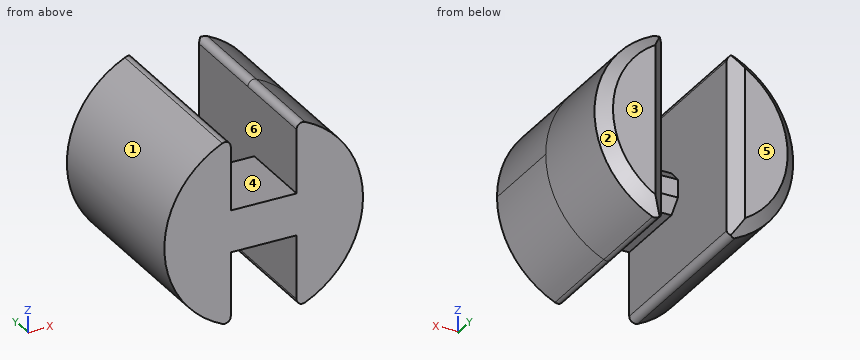
```python
from build123d import *

# Parameters (mm, degrees)
SKETCH1_W           = 2.75
SKETCH1_H           = 1.75
BOSS_EXTRUDE1_DEPTH = 3.75
BOSS_EXTRUDE2_DEPTH = 4.25
FILLET1_R           = 0.25
CHAMFER1_SIZE       = 0.5


with BuildPart() as part:
    # Sketch1 → Boss-Extrude1 (new body)
    with BuildSketch(Plane(origin=(0, 0, 0), x_dir=(1, 0, 0), z_dir=(0, 1, 0))):
        with BuildLine():
            Line((-1.375, 0.875), (-1.375, 3.915593825))
            ThreePointArc((-1.375, 3.915593825), (-4.15, 0), (-1.375, -3.915593825))
            Line((-1.375, -3.915593825), (-1.375, -0.875))
            Line((-1.375, -0.875), (-1.375, 0.875))
        make_face()
        with BuildLine():
            ThreePointArc((4.15, 0), (3.385908298, 2.399609343), (1.375, 3.915593825))
            Line((1.375, 3.915593825), (1.375, 0.875))
            Line((1.375, 0.875), (1.375, -0.875))
            Line((1.375, -0.875), (1.375, -3.915593825))
            ThreePointArc((1.375, -3.915593825), (3.385908298, -2.399609343), (4.15, 0))
        make_face()
        Rectangle(SKETCH1_W, SKETCH1_H)
    extrude(amount=BOSS_EXTRUDE1_DEPTH)

    # Sketch2 → Boss-Extrude2 (add)
    with BuildSketch(Plane(origin=(0, 3.75, 0), x_dir=(1, 0, 0), z_dir=(0, 1, 0))):
        with BuildLine():
            Line((1.375, -0.875), (1.375, 0.875))
            Line((1.375, 0.875), (1.375, 3.915593825))
            ThreePointArc((1.375, 3.915593825), (4.15, 0), (1.375, -3.915593825))
            Line((1.375, -3.915593825), (1.375, -0.875))
        make_face()
        with BuildLine():
            Line((-1.375, 0.875), (-1.375, -0.875))
            Line((-1.375, -0.875), (-1.375, -3.915593825))
            ThreePointArc((-1.375, -3.915593825), (-4.15, 0), (-1.375, 3.915593825))
            Line((-1.375, 3.915593825), (-1.375, 0.875))
        make_face()
    extrude(amount=BOSS_EXTRUDE2_DEPTH)

    # Fillet1
    fillet1_edges = [part.edges().sort_by_distance(p)[0] for p in [
        (1.375, 4, -3.915593825),
        (1.375, 4, 3.915593825),
        (-1.375, 4, 3.915593825),
        (-1.375, 4, -3.915593825),
    ]]
    fillet(fillet1_edges, radius=FILLET1_R)

    # Chamfer1
    # the kernel refuses this chamfer: 0.5 mm, written as the material it takes off along each edge
    with BuildSketch(Plane(origin=(0, 8, 0), x_dir=(0.11938589143460555, 0, -0.99284792839909), z_dir=(-0.99284792839909, 0, -0.11938589143460555))) as chamfer1_piece_1:
        Polygon((4.15, CHAMFER1_SIZE), (4.15 - CHAMFER1_SIZE, 0), (4.15, 0), align=None)
    revolve(axis=Axis((0, 8, 0), (0, -1, 0)), revolution_arc=166.286676069, mode=Mode.SUBTRACT)
    with BuildSketch(Plane(origin=(1.375, 8, 4.831172931), x_dir=(-0.02749587661058651, -0.9996219169112968, 0), z_dir=(0, 0, -1)), Plane(origin=(-1.375, 8, -4.831172931), x_dir=(0.02749587661058651, -0.9996219169112968, 0), z_dir=(0, 0, 1))) as chamfer1_piece_2:
        Polygon((CHAMFER1_SIZE * 0.999621916911, -CHAMFER1_SIZE * 0.0274958766106), (-CHAMFER1_SIZE * 0.0274958766106, -CHAMFER1_SIZE * 0.999621916911), (0, 0), align=None)
    extrude(amount=9.662345862, mode=Mode.SUBTRACT)
    with BuildSketch(Plane(origin=(0, 8, 0), x_dir=(-0.11938589143460458, 0, 0.9928479283990902), z_dir=(0.9928479283990902, 0, 0.11938589143460458))) as chamfer1_piece_3:
        Polygon((4.15 - CHAMFER1_SIZE, 0), (4.15, CHAMFER1_SIZE), (4.15, 0), align=None)
    revolve(axis=Axis((0, 8, 0), (0, -1, 0)), revolution_arc=166.286676069, mode=Mode.SUBTRACT)
    with BuildSketch(Plane(origin=(-1.375, 3.75, 0.875), x_dir=(0, -0.9996219169112968, 0.02749587661058627), z_dir=(1, 0, 0))) as chamfer1_piece_4:
        Polygon((CHAMFER1_SIZE * 0.999621916911, CHAMFER1_SIZE * 0.0274958766106), (-CHAMFER1_SIZE * 0.0274958766106, CHAMFER1_SIZE * 0.999621916911), (0, 0), align=None)
    extrude(amount=2.75, mode=Mode.SUBTRACT)
    with BuildSketch(Plane(origin=(1.375, 3.75, -0.875), x_dir=(0, 0.027495876610586487, 0.9996219169112968), z_dir=(-1, 0, 0))) as chamfer1_piece_5:
        Polygon((CHAMFER1_SIZE * 0.999621916911, -CHAMFER1_SIZE * 0.0274958766106), (-CHAMFER1_SIZE * 0.0274958766106, -CHAMFER1_SIZE * 0.999621916911), (0, 0), align=None)
    extrude(amount=2.75, mode=Mode.SUBTRACT)


solid = part.part
```
Check sheet for the modelled part. Datum: model origin and axes. Units: mm. Face numbers are marked on the shaded views. A direction names the side the tool comes from. Round coordinates to 2 decimals unless told otherwise and drop trailing zeros. Loops run counter-clockwise (first coordinate to the right, second up) from the corner with the lowest first, then second, coordinate; pieces in that order, holes last. Notation, with made-up numbers: (22, 36) - (67, 36) arc R19 ccw to (67, 59) - close; hole circle Ø7 at (-31.75, 61.5). An arc over 180 degrees is marked (long way). Answer as a JSON object with one key per item and string values. Group by question number.
Q1. Gauge pin test, flat ends, axial feed: P1, Ø3, axis at x = 0, y = 1, coming from the +Z side; P2, Ø0.8, axis at x = 0.5, z = 0, coming from the +Y side; P3, Ø0.8, axis at x = 0, y = 2, coming from the -Z side (3 decimals). Record the tip position at first contact, or that the pin passes through.
Q2. Sectioned sample at B-B, the plane x = -0.75. Enter the section's corners in (y, z) (3 decimals).
Q3. Scan lines: line 1 along X through (y, z) = (5, -1.5) (3 decimals); line 2 along X through (y, z) = (0.5, 1.75) (3 decimals); line 3 along Y through (x, z) = (1.5, -3) (3 decimals). Record each from-to range of solid material in increasing order. Write a range as [from, to].
Q4. Sectioned sample at C-C, the plane y = 2. Enter the section's corners in (x, z) (3 decimals).
Q5. Sectioned sample at A-A, the plane y = 5. Enter the section's corners in (x, z) (3 decimals), plus the area to 3 significant figures.
Q6. Set-up check for the marked faces 5 and 6: record each of +Z, -Z, +X, -X, +Y, -Y from which the full face is reachable in a straight line by a thin tool's end or side.
Q7. Mould release check, pull along X, two halves, no side actions. Record for the marked faces 1, 2, 3 and 4: released by +X, released by -X, zero draft, split by the parting line, or undercut.
Solution:
{
 "1": {"P1": "stops at z = 3.76", "P2": "stops at y = 3.75", "P3": "stops at z = -0.875"},
 "2": {"outline": "(0, -0.875) - (3.25, -0.875) - (3.75, -0.375) - (3.75, 0.375) - (3.25, 0.875) - (0, 0.875) - close"},
 "3": {"line 1": "x = [-3.869, -1.375], [1.375, 3.869]", "line 2": "x = [-3.763, -1.375], [1.375, 3.763]", "line 3": "y = [0, 7.625]"},
 "4": {"outline": "(-1.729, -3.773) arc R0.25 ccw to (-1.375, -3.545) - (-1.375, -0.875) - (1.375, -0.875) - (1.375, -3.545) arc R0.25 ccw to (1.729, -3.773) arc R4.15 ccw to (1.729, 3.773) arc R0.25 ccw to (1.375, 3.545) - (1.375, 0.875) - (-1.375, 0.875) - (-1.375, 3.545) arc R0.25 ccw to (-1.729, 3.773) arc R4.15 ccw to start"},
 "5": {"outline": "(-1.729, -3.773) arc R0.25 ccw to (-1.375, -3.545) - (-1.375, 3.545) arc R0.25 ccw to (-1.729, 3.773) arc R4.15 ccw to start; (1.375, -3.545) arc R0.25 ccw to (1.729, -3.773) arc R4.15 ccw to (1.729, 3.773) arc R0.25 ccw to (1.375, 3.545) - close", "area": "31.6 mm²"},
 "6": {"face 5": "+Z, -Z, +X, -X, +Y", "face 6": "+Y"},
 "7": {"face 1": "released by -X", "face 2": "released by +X", "face 3": "zero draft", "face 4": "undercut"}
}
